```python
from build123d import *

# Parameters (mm, degrees)
F0_W     = 12.7
F0_H     = 5.08
F1_DEPTH = 7.62
F2_W     = 12.7
F2_H     = 5.08
F3_DEPTH = 12.7
F4_R     = 5.55625
F5_DEPTH = 25.4
F6_R     = 5.08


with BuildPart() as f1:
    # F0 (on Top) → F1 (new body)
    with BuildSketch(Plane.XY):
        with Locations((-86.055439, 58.905405)):
            Rectangle(F0_W, F0_H)
    extrude(amount=F1_DEPTH)

    # F2 (on face) → F3 (join)
    with BuildSketch(Plane.XY.offset(7.62)):
        with Locations((-86.055439, 58.905405)):
            Rectangle(F2_W, F2_H)
    extrude(amount=F3_DEPTH)

    # F4 (on face) → F5 (cut)
    with BuildSketch(Plane.XZ.offset(-56.365405)):
        with Locations((-86.055439, 13.97)):
            Circle(F4_R)
    extrude(amount=-F5_DEPTH, mode=Mode.SUBTRACT)

    # F6
    f6_edges = [f1.edges().sort_by_distance(p)[0] for p in [
        (-92.405439, 58.905405, 20.32),
        (-79.705439, 58.905405, 20.32),
    ]]
    fillet(f6_edges, radius=F6_R)


solid = f1.part
```
For this review, take the finished solid that the model builds, in its own axes (mm). Coordinates: 2 decimals unless noted, no trailing zeros. Order: outer loops, then holes, each group sorted by start corner. A loop starts at its lowest first (then second) coordinate and runs counter-clockwise, first axis right, second up. Notation, with made-up numbers: (82, -34.75) -> (96, -34.75) arc R31 cw to (96, -2.75) -> close; hole circle Ø10 at (69, -26.75). An arc over 180 degrees is marked (long way). Answer as CSV lines item,"result".
Q1. Clearance check with flat-ended pins moving along their axes: pin 1 Ø1.5 at (x, z) = (-82, 15) entering from +Y; pin 2 Ø1 at (x, y) = (-83, 57.5) entering from +Z. State where each tip first meets the part, or that it passes through.
Model answer:
pin 1,"passes through"
pin 2,"stops at z = 20.15"
Q2. Wall thickness on line 1 along Z through (x, y) = (-85.75, 60.1); line 2 along Z through (x, y) = (-88.25, 59.2); line 3 along X through (y, z) = (58.6, 13): over which ranges is each line inside the solid? List them lowest first. Write a range as [from, to].
Model answer:
line 1,"z = [0, 8.42], [19.52, 20.32]"
line 2,"z = [0, 8.87], [19.07, 20.24]"
line 3,"x = [-92.41, -91.53], [-80.58, -79.71]"
Q3. Draft analysis for pull direction X (two halves, no side actions). For faces 1 (the face through (-92.405, 59, 8)), 2 (the face through (-80.756, 58.87, 15.639)), 3 (the face through (-79.705, 59, 8)), state which applies: released by +X, released by -X, zero draft, split by the parting line, or undercut.
Model answer:
face 1,"released by -X"
face 2,"undercut"
face 3,"released by +X"
Q4. We need section C-C (x = -82.5). State the section outline as (y, z) points.
Model answer:
outline,"(56.37, 0) -> (61.45, 0) -> (61.45, 9.7) -> (56.37, 9.7) -> close; (56.37, 18.24) -> (61.45, 18.24) -> (61.45, 19.78) -> (56.37, 19.78) -> close"
Q5. We need section A-A (z = 13.97). State the section outline as (x, y) points, plus the area to 3 significant figures.
Model answer:
outline,"(-92.41, 56.37) -> (-91.61, 56.37) -> (-91.61, 61.45) -> (-92.41, 61.45) -> close; (-80.5, 56.37) -> (-79.71, 56.37) -> (-79.71, 61.45) -> (-80.5, 61.45) -> close"
area,"8.06 mm2"
Q6. We need section B-B (y = 61.05). State the section outline as (x, z) points.
Model answer:
outline,"(-92.41, 0) -> (-79.71, 0) -> (-79.71, 15.24) arc R5.08 ccw to (-84.79, 20.32) -> (-87.33, 20.32) arc R5.08 ccw to (-92.41, 15.24) -> close; hole circle Ø11.11 at (-86.06, 13.97)"
